```python
from build123d import *

# Parameters (mm, degrees)
BOSS_EXTRUDE1_DEPTH        = 489.54
BOSS_EXTRUDE1_DEPTH_BACK   = 430
SKETCH2_W                  = 30
SKETCH2_H                  = 30
BOSS_EXTRUDE1_2_DEPTH      = 489.54
BOSS_EXTRUDE1_2_DEPTH_BACK = 430
SKETCH3_W                  = 30
SKETCH3_H                  = 30
BOSS_EXTRUDE2_DEPTH        = 430
BOSS_EXTRUDE2_2_DEPTH      = 430
BOSS_EXTRUDE3_DEPTH        = 30
BOSS_EXTRUDE4_DEPTH        = 130
CUT_EXTRUDE2_REACH         = 675.85
CUT_EXTRUDE2_END_RADIUS    = 915
FILLET1_R                  = 10
SKETCH8_W                  = 390
SKETCH8_H                  = 49.54
CUT_EXTRUDE3_DEPTH         = 674.850437188


with BuildPart() as part:
    # Sketch2 → Boss-Extrude1 (new, two sides: drawn at the far end of the back side and taken through both)
    with BuildSketch(Plane(origin=(0, 0, 0), x_dir=(1, 0, 0), z_dir=(0, 1, 0)).offset(-BOSS_EXTRUDE1_DEPTH_BACK)):
        with Locations((-180, -195)):
            Rectangle(SKETCH2_W, SKETCH2_H)
    extrude(amount=BOSS_EXTRUDE1_DEPTH + BOSS_EXTRUDE1_DEPTH_BACK)



with BuildPart() as body_2:
    # Sketch2 → Boss-Extrude1 2 (new, two sides: drawn at the far end of the back side and taken through both)
    with BuildSketch(Plane(origin=(0, 0, 0), x_dir=(1, 0, 0), z_dir=(0, 1, 0)).offset(-BOSS_EXTRUDE1_2_DEPTH_BACK)):
        with Locations((180, -195)):
            Rectangle(SKETCH2_W, SKETCH2_H)
    extrude(amount=BOSS_EXTRUDE1_2_DEPTH + BOSS_EXTRUDE1_2_DEPTH_BACK)


with BuildPart() as body_3:
    # Sketch3 → Boss-Extrude2 (new body)
    with BuildSketch(Plane(origin=(0, 0, 0), x_dir=(1, 0, 0), z_dir=(0, 1, 0))):
        with Locations((-180, 195)):
            Rectangle(SKETCH3_W, SKETCH3_H)
    extrude(amount=-BOSS_EXTRUDE2_DEPTH)


with BuildPart() as body_4:
    # Sketch3 → Boss-Extrude2 2 (new body)
    with BuildSketch(Plane(origin=(0, 0, 0), x_dir=(1, 0, 0), z_dir=(0, 1, 0))):
        with Locations((180, 195)):
            Rectangle(SKETCH3_W, SKETCH3_H)
    extrude(amount=-BOSS_EXTRUDE2_2_DEPTH)


with BuildPart() as part_1:
    add(part.part)

    add(body_2.part)  # Boss-Extrude3 merges body 2

    add(body_3.part)  # Boss-Extrude3 merges body 3

    add(body_4.part)  # Boss-Extrude3 merges body 4
    # Sketch4 → Boss-Extrude3 (add)
    with BuildSketch(Plane(origin=(0, 0, 0), x_dir=(1, 0, 0), z_dir=(0, 1, 0))):
        Polygon((-165, 210), (165, 210), (165, 180), (195, 180), (195, -180), (165, -180), (165, -210), (-165, -210), (-165, -180), (-195, -180), (-195, 180), (-165, 180), align=None)
    extrude(amount=-BOSS_EXTRUDE3_DEPTH)

    # Sketch5 → Boss-Extrude4 (add)
    with BuildSketch(Plane(origin=(0, 489.54, 0), x_dir=(1, 0, 0), z_dir=(0, 1, 0))):
        with BuildLine():
            Line((-165, -180), (-165, -210))
            Line((-165, -210), (165, -210))
            Line((165, -210), (165, -180))
            ThreePointArc((165, -180), (0, -195), (-165, -180))
        make_face()
    extrude(amount=-BOSS_EXTRUDE4_DEPTH)

    # Cut-Extrude2: up to this cylinder (the profile starts outside it)
    cut_extrude2_end = Plane(origin=(0, 479.936128, -720), z_dir=(0, 1, 0)) * Cylinder(CUT_EXTRUDE2_END_RADIUS, 3182.7, mode=Mode.PRIVATE)
    # Sketch7 → Cut-Extrude2 (cut, up to the surface)
    with BuildSketch(Plane.XY.offset(210), mode=Mode.PRIVATE) as cut_extrude2_sk1:
        with BuildLine():
            Line((75, 489.54), (-75, 489.54))
            Line((-75, 489.54), (-63, 473.54))
            ThreePointArc((-63, 473.54), (-59.472135955, 470.59572809), (-55, 469.54))
            Line((-55, 469.54), (55, 469.54))
            ThreePointArc((55, 469.54), (59.472135955, 470.59572809), (63, 473.54))
            Line((63, 473.54), (75, 489.54))
        make_face()
    cut_extrude2_tool1 = extrude(cut_extrude2_sk1.sketch, amount=-CUT_EXTRUDE2_REACH, mode=Mode.PRIVATE) - cut_extrude2_end
    add(cut_extrude2_tool1.solids().sort_by_distance((0, 479.936128, 210))[0], mode=Mode.SUBTRACT)

    # Fillet1
    fillet1_edges = [part_1.edges().sort_by_distance(p)[0] for p in [
        (75, 489.54, 200.960524607),
        (-75, 489.54, 200.960524607),
    ]]
    fillet(fillet1_edges, radius=FILLET1_R)

    # Sketch8 → Cut-Extrude3 (cut, through all)
    with BuildSketch(Plane.XY.offset(210)):
        with Locations((0, -405.23)):
            Rectangle(SKETCH8_W, SKETCH8_H)
    extrude(amount=-CUT_EXTRUDE3_DEPTH, mode=Mode.SUBTRACT)


solid = part_1.part
```
Check sheet for the modelled part. Datum: model origin and axes. Units: mm. A direction names the side the tool comes from. Coordinates: 2 decimals unless noted, no trailing zeros. Order: outer loops, then holes, each group sorted by start corner. A loop starts at its lowest first (then second) coordinate and runs counter-clockwise, first axis right, second up. Notation, with made-up numbers: M 47,82 L 86,82 A20 ccw 86,96 Z; hole C 45.25,-15 d5. An arc over 180 degrees is marked long. Write each question's results on one line, items separated by ' | '. Start each with the question number.
1. Access from +Z, -Z, +X, -X, +Y, -Y to the whole of each face (thin tool, end or side, straight path). Record for faces 1 (the face through (180, 241, 180)), 2 (the face through (-1, 469.54, 202)), 3 (the face through (-165, -208, 195)), 4 (the face through (-180, -380.46, 195)), 5 (the face through (-2, 359.54, 198)).
2. Material ranges on probe 1 along Z at (x, y) = (-171, -54); probe 2 along Y at (x, z) = (111.5, 192); probe 3 along Y at (x, z) = (126, 180), recorded low to high.
3. Mould release check, pull along Z, two halves, no side actions. Record for faces 6 (the face through (-30, -20, -210)), 7 (the face through (-180, -203, -180)), 8 (the face through (-180, -208, 180)), 9 (the face through (-195, -8, 63)): +Z half, -Z half, draft (parallel to the pull), parting line (faces both ways), or undercut.
4. Cross-section at D-D on z = -105. Record the cut outline in (x, y), and give its area (3 significant figures).
5. Cross-section at C-C on y = -90.5. Record the cut outline in (x, z), and give its area (3 significant figures).
6. Cross-section at A-A on y = 309.5. Record the cut outline in (x, z).
7. Go/stop test with flat-tipped pins: P1, Ø15, axis at x = 183.5, y = 238.5, coming from the -Z side; P2, Ø8, axis at x = -52.5, z = -108.5, coming from the +Y side; P3, Ø6, axis at x = -97, z = 119.5, coming from the -Y side. Record where each tip stops, or that it passes through.
8. Cross-section at B-B on x = 0. Record the cut outline in (y, z).
Checks:
1) face 1: -Z, +X, -X, +Y | face 2: +Z, -Z, +Y | face 3: +Z, -Z, -Y | face 4: +Z, -Z, +X, -X, -Y | face 5: +Z, -Z
2) probe 1: z = -210 to -180, 180 to 210 | probe 2: y = -30 to 0, 359.54 to 489.54 | probe 3: y = -30 to 0
3) face 6: -Z half | face 7: undercut | face 8: undercut | face 9: draft
4) outline: M -195,-30 L 195,-30 L 195,0 L -195,0 Z | area: 11,700 mm²
5) outline: M -195,-210 L -165,-210 L -165,-180 L -195,-180 Z; M -195,180 L -165,180 L -165,210 L -195,210 Z; M 165,-210 L 195,-210 L 195,-180 L 165,-180 Z; M 165,180 L 195,180 L 195,210 L 165,210 Z | area: 3,600 mm²
6) outline: M -195,180 L -165,180 L -165,210 L -195,210 Z; M 165,180 L 195,180 L 195,210 L 165,210 Z
7) P1: stops at z = 180 | P2: stops at y = 0 | P3: stops at y = -30
8) outline: M -30,-210 L 0,-210 L 0,210 L -30,210 Z; M 359.54,195 L 469.54,195 L 469.54,210 L 359.54,210 Z
